Geometry: final body of the model. Coordinates: model frame, mm. A direction names the side the tool comes from. Give positions to 0.01 mm unless a question says otherwise; leave off trailing zeros. Write each loop counter-clockwise with the first axis right and the second up, starting at its lowest first coordinate (ties: lowest second). Pieces come first, ordered by that corner, then holes.
```python
from build123d import *

# Parameters (mm, degrees)
EXTRUDE031_DEPTH = 5
SKETCH021_R      = 1.125
EXTRUDE005_DEPTH = 5
SKETCH020_W      = 8
SKETCH020_H      = 25.5
SKETCH020_R      = 1.625
EXTRUDE004_DEPTH = 5
SKETCH019_R      = 1.125
EXTRUDE003_DEPTH = 5
SKETCH093_W      = 82
SKETCH093_H      = 72
SKETCH093_R      = 1.625
EXTRUDE030_DEPTH = 4.5


with BuildPart() as obj1:
    # Sketch094 → Extrude031 (new body)
    with BuildSketch(Plane.XY):
        with BuildLine():
            ThreePointArc((-7.5, -283.5), (-12.5, -288.5), (-7.5, -293.5))
            Line((-7.5, -293.5), (0, -293.5))
            ThreePointArc((0, -293.5), (5, -288.5), (0, -283.5))
            Line((0, -283.5), (-7.5, -283.5))
        make_face()
    extrude(amount=EXTRUDE031_DEPTH)


with BuildPart() as obj1_1:
    # Extrude031 placement: moved
    add(obj1.part.moved(Location((0, 0, -309.75))))


with BuildPart() as obj2:
    # Sketch021 (on Extrude) → Extrude005 (new body)
    with BuildSketch(Plane.XZ):
        Polygon((-25, -309), (-25, -301), (16.5, -301), (16.5, -263), (24.5, -263), (24.5, -309), align=None)
        with Locations((-20.4, -304.4)):
            Circle(SKETCH021_R, mode=Mode.SUBTRACT)
        with Locations((20.4, -267.6)):
            Circle(SKETCH021_R, mode=Mode.SUBTRACT)
    extrude(amount=EXTRUDE005_DEPTH)


with BuildPart() as obj2_1:
    # Extrude005 placement: moved
    add(obj2.part.moved(Location((0, -262.5, 0))))


with BuildPart() as gpshold:
    # Sketch020 → Extrude004 (new body)
    with BuildSketch(Plane.XY.offset(-263)):
        with Locations((15, -294.25)):
            Rectangle(SKETCH020_W, SKETCH020_H)
        with Locations((15, -284.1)):
            Circle(SKETCH020_R, mode=Mode.SUBTRACT)
        with Locations((15, -304.5)):
            Circle(SKETCH020_R, mode=Mode.SUBTRACT)
    extrude(amount=EXTRUDE004_DEPTH)


with BuildPart() as obj3:
    # Sketch019 → Extrude003 (new body)
    with BuildSketch(Plane.XZ.offset(295)):
        Polygon((28, -309), (28, -301), (19, -301), (19, -263), (11, -263), (11, -301), (-13, -301), (-13, -284), (-19, -284), (-19, -309), align=None)
        with Locations((-15.96, -286.8)):
            Circle(SKETCH019_R, mode=Mode.SUBTRACT)
        with Locations((-0.15, -304.37)):
            Circle(SKETCH019_R, mode=Mode.SUBTRACT)
        with Locations((20.15, -304.37)):
            Circle(SKETCH019_R, mode=Mode.SUBTRACT)
        with Locations((16.04, -270.55)):
            Circle(SKETCH019_R, mode=Mode.SUBTRACT)
    extrude(amount=EXTRUDE003_DEPTH)


with BuildPart() as base012:
    # Sketch093 → Extrude030 (new body)
    with BuildSketch(Plane.XY):
        with Locations((0, -285)):
            Rectangle(SKETCH093_W, SKETCH093_H)
        with Locations((-35, -315)):
            Circle(SKETCH093_R, mode=Mode.SUBTRACT)
        with Locations((35, -315)):
            Circle(SKETCH093_R, mode=Mode.SUBTRACT)
        with Locations((35, -255)):
            Circle(SKETCH093_R, mode=Mode.SUBTRACT)
        with Locations((-35, -255)):
            Circle(SKETCH093_R, mode=Mode.SUBTRACT)
        with BuildLine():
            ThreePointArc((-3.658125, -285.3), (-12.5, -288.5), (-3.658125, -291.7))
            Line((-0.399218, -291.675), (-3.658125, -291.7))
            ThreePointArc((-0.399218, -291.675), (3.2, -288.5), (-0.399218, -285.325))
            Line((-0.399218, -285.325), (-3.658125, -285.3))
        make_face(mode=Mode.SUBTRACT)
        with BuildLine():
            ThreePointArc((-2, -253), (-4, -255), (-2, -257))
            Line((2, -258), (-2, -257))
            ThreePointArc((2, -258), (5, -255), (2, -252))
            Line((-2, -253), (2, -252))
        make_face(mode=Mode.SUBTRACT)
    extrude(amount=EXTRUDE030_DEPTH)


with BuildPart() as base012_1:
    # Extrude030 placement: moved
    add(base012.part.moved(Location((0, 0, -313.5))))

    # Fusion078: union obj2, gpsHold, obj3
    add(obj2_1.part)
    add(gpshold.part)
    add(obj3.part)

    # Cut035: cut obj1
    add(obj1_1.part, mode=Mode.SUBTRACT)


solid = base012_1.part
```
Item 1: Section D-D, the plane y = -266. Return the cut outline in (x, z) (3 decimals).
Found:
outline: (-41, -313.5) - (41, -313.5) - (41, -309) - (24.5, -309) - (24.5, -263) - (16.5, -263) - (16.5, -301) - (-25, -301) - (-25, -309) - (-41, -309) - close; hole circle Ø2.25 at (-20.4, -304.4); hole circle Ø2.25 at (20.4, -267.6)
Item 2: Pull-direction query (Z, two-part tool) for faces 5 (the face through (-20.546, -264.965, -303.285)), 6 (the face through (0, -252.5, -311.3)), 7 (the face through (19.91, -297.46, -305.47)), 8 (the face through (24, -297, -301)); classes: +Z half, -Z half, draft (parallel to the pull), parting line (faces both ways), or undercut.
Found:
face 5: undercut
face 6: draft
face 7: undercut
face 8: +Z half
Item 3: Pin query (flat end, axial travel): pin 1 Ø5.5 at (x, y) = (19, -265) entering from +Z; pin 2 Ø8 at (y, z) = (-297, -297.5) entering from +X; pin 3 Ø13 at (y, z) = (-290, -271) entering from +X. Return the tip coordinate at first contact, or that it passes through.
Found:
pin 1: stops at z = -263
pin 2: stops at x = 28
pin 3: stops at x = 19
Item 4: Section A-A, the plane z = -286.8. Return the cut outline in (x, y) (3 decimals).
Found:
outline: (-19, -300) - (-17.085, -300) - (-17.085, -295) - (-19, -295) - close; (-14.835, -300) - (-13, -300) - (-13, -295) - (-14.835, -295) - close; (11, -300) - (19, -300) - (19, -295) - (11, -295) - close; (16.5, -267.5) - (24.5, -267.5) - (24.5, -262.5) - (16.5, -262.5) - close
Item 5: Line query: L1, parallel to Y at x = 15, z = -261.65 (3 decimals); L2, parallel to Y at x = 35, z = -310 (3 decimals); L3, parallel to Z at x = -20.5, y = -266.5. Output: solid intervals per line, ascending.
Found:
L1: y = -307 to -306.125, -302.875 to -285.725, -282.475 to -281.5
L2: y = -321 to -316.625, -313.375 to -256.625, -253.375 to -249
L3: z = -313.5 to -305.52, -303.28 to -301
Item 6: Reachability of faces 1 (the face through (16.5, -265, -282)), 2 (the face through (15.8, -297.46, -271.65)), 3 (the face through (-19, -297, -296)), 4 (the face through (11, -296, -273)) from +Z, -Z, +X, -X, +Y, -Y: full face, straight path, thin tool, end or side. Return the list, or none.
Found:
face 1: +Z, -X, +Y
face 2: -Y
face 3: +Z, -X, -Y
face 4: +Z, +Y, -Y
Item 7: Section C-C, the plane x = -20.4. Return the cut outline in (y, z) (3 decimals).
Found:
outline: (-321, -313.5) - (-249, -313.5) - (-249, -309) - (-262.5, -309) - (-262.5, -305.525) - (-267.5, -305.525) - (-267.5, -309) - (-321, -309) - close; (-267.5, -303.275) - (-262.5, -303.275) - (-262.5, -301) - (-267.5, -301) - close
Item 8: Section B-B, the plane z = -296. Return the cut outline in (x, y).
Found:
outline: (-19, -300) - (-13, -300) - (-13, -295) - (-19, -295) - close; (11, -300) - (19, -300) - (19, -295) - (11, -295) - close; (16.5, -267.5) - (24.5, -267.5) - (24.5, -262.5) - (16.5, -262.5) - close
